from build123d import *

# Parameters (mm, degrees)
SKICA1_W                = 6
SKICA1_H                = 3.2
P_IDAT_VYSUNUT_M1_DEPTH = 3.4
SKICA2_W                = 3
SKICA2_H                = 1.6
P_IDAT_VYSUNUT_M2_DEPTH = 1
SKICA3_W                = 0.7
SKICA3_H                = 2
P_IDAT_VYSUNUT_M3_DEPTH = 0.3


with BuildPart() as part:
    # Skica1 → Přidat vysunutím1 (new body)
    with BuildSketch(Plane.XY):
        Rectangle(SKICA1_W, SKICA1_H)
    extrude(amount=P_IDAT_VYSUNUT_M1_DEPTH)

    # Skica2 → Přidat vysunutím2 (add)
    with BuildSketch(Plane(origin=(0, 1.6, 0), x_dir=(1, 0, 0), z_dir=(0, 1, 0))):
        with Locations((0, -1.7)):
            Rectangle(SKICA2_W, SKICA2_H)
    extrude(amount=P_IDAT_VYSUNUT_M2_DEPTH)

    # Skica3 → Přidat vysunutím3 (add)
    with BuildSketch(Plane(origin=(0, 1.6, 0), x_dir=(1, 0, 0), z_dir=(0, 1, 0))):
        with Locations((-2.35, -1.7)):
            Rectangle(SKICA3_W, SKICA3_H)
        with Locations((2.35, -1.7)):
            Rectangle(SKICA3_W, SKICA3_H)
    extrude(amount=P_IDAT_VYSUNUT_M3_DEPTH)


solid = part.part
Input: part model. Units: mm. Frame: model coordinates. A direction names the side the tool comes from. Round coordinates to 2 decimals unless told otherwise and drop trailing zeros. Order: outer loops, then holes, each group sorted by start corner. A loop starts at its lowest first (then second) coordinate and runs counter-clockwise, first axis right, second up. Notation, with made-up numbers: (19.5, 4) - (42.5, 4) arc R25 cw to (42.5, 33) - close; hole circle Ø11 at (77, -17). An arc over 180 degrees is marked (long way). Answer as a JSON object with one key per item and string values. Group by question number.
(1) Reachability of faces 1 (the face through (0, 2, 2.5)), 2 (the face through (1.5, 2, 2)), 3 (the face through (-3, 0, 2)) from +Z, -Z, +X, -X, +Y, -Y: full face, straight path, thin tool, end or side. Return the list, or none.
(2) Material intervals for probe 1 along X at (y, z) = (1.7, 1.8); probe 2 along Y at (x, z) = (1.7, 1.15); probe 3 along Z at (x, y) = (1.05, 1.7), sorted ascending. Write a range as from..to.
(3) Cut plane D-D (z = 2.8). Return loops of the section in (x, y).
(4) Cut plane A-A (x = -0.65). Return loops of the section in (y, z).
(5) Pin query (flat end, axial travel): P1, Ø0.5, axis at y = 2, z = 2, coming from the +X side; P2, Ø0.8, axis at x = 2, z = 2, coming from the +Y side. Return the tip coordinate at first contact, or that it passes through.
(6) Cut plane B-B (z = 1.35). Return loops of the section in (x, y).
(7) Cut plane C-C (x = -2.55). Return loops of the section in (y, z).
(8) Draft query along X for faces 4 (the face through (3, 0, 2)), 5 (the face through (0, 2.6, 2)), 6 (the face through (0, 2, 0.9)). Return one class per face: released by +X, released by -X, zero draft, split by the parting line, or undercut.
Here are the results:
{
 "1": {"face 1": "+Z, +Y", "face 2": "+Z, -Z, +Y", "face 3": "+Z, -Z, -X, +Y, -Y"},
 "2": {"probe 1": "x = -2.7..-2, -1.5..1.5, 2..2.7", "probe 2": "y = -1.6..1.6", "probe 3": "z = 0.9..2.5"},
 "3": {"outline": "(-3, -1.6) - (3, -1.6) - (3, 1.6) - (-3, 1.6) - close"},
 "4": {"outline": "(-1.6, 0) - (1.6, 0) - (1.6, 0.9) - (2.6, 0.9) - (2.6, 2.5) - (1.6, 2.5) - (1.6, 3.4) - (-1.6, 3.4) - close"},
 "5": {"P1": "stops at x = 2.7", "P2": "stops at y = 1.9"},
 "6": {"outline": "(-3, -1.6) - (3, -1.6) - (3, 1.6) - (2.7, 1.6) - (2.7, 1.9) - (2, 1.9) - (2, 1.6) - (1.5, 1.6) - (1.5, 2.6) - (-1.5, 2.6) - (-1.5, 1.6) - (-2, 1.6) - (-2, 1.9) - (-2.7, 1.9) - (-2.7, 1.6) - (-3, 1.6) - close"},
 "7": {"outline": "(-1.6, 0) - (1.6, 0) - (1.6, 0.7) - (1.9, 0.7) - (1.9, 2.7) - (1.6, 2.7) - (1.6, 3.4) - (-1.6, 3.4) - close"},
 "8": {"face 4": "released by +X", "face 5": "zero draft", "face 6": "undercut"}
}
